```python
from build123d import *

# Parameters (mm, degrees)
BOSS_EXTRUDE1_DEPTH  = 3.175
BOSS_EXTRUDE2_DEPTH  = 3.175
M4_CLEARANCE_HOLE1_D = 4.5
SKETCH7_R            = 1.7
CUT_EXTRUDE1_DEPTH   = 4.175


with BuildPart() as part:
    # Sketch1 → Boss-Extrude1 (new body)
    with BuildSketch(Plane(origin=(0, 0, 0), x_dir=(1, 0, 0), z_dir=(0, 1, 0))):
        with BuildLine():
            ThreePointArc((0, 85), (-61.668691787, 60.61327124), (-89.979209979, 0.644490644))
            Line((-89.979209979, 0.644490644), (-69.92561449, 0.644490644))
            ThreePointArc((-69.92561449, 0.644490644), (-47.516373878, 46.462349638), (0, 65))
            Line((0, 65), (0, 85))
        make_face()
    extrude(amount=BOSS_EXTRUDE1_DEPTH)

    # Sketch2 → Boss-Extrude2 (add)
    with BuildSketch(Plane(origin=(0, 3.175, 0), x_dir=(1, 0, 0), z_dir=(0, 1, 0))):
        with BuildLine():
            Line((-89.979209979, 20.644490644), (-89.979209979, 0.644490644))
            ThreePointArc((-89.979209979, 0.644490644), (-88.75145348, 10.745821604), (-86.393355856, 20.644490644))
            Line((-86.393355856, 20.644490644), (-89.979209979, 20.644490644))
        make_face()
        with BuildLine():
            Line((-35, 85), (-35, 77.929830117))
            ThreePointArc((-35, 77.929830117), (-17.853482169, 83.214784737), (0, 85))
            Line((0, 85), (-35, 85))
        make_face()
    extrude(amount=-BOSS_EXTRUDE2_DEPTH)

    # M4 Clearance Hole1 (through all)
    with Locations(Plane.XZ):
        with Locations((-27.5, -70), (-7.5, -80), (-27.5, -80), (-7.5, -70)):
            Hole(M4_CLEARANCE_HOLE1_D / 2)

    # Sketch7 → Cut-Extrude1 (cut, through all)
    with BuildSketch(Plane.XZ):
        with Locations((-70.979209979, -15.644490644)):
            Circle(SKETCH7_R)
        with Locations((-85.979209979, -15.644490644)):
            Circle(SKETCH7_R)
        with Locations((-85.979209979, -5.644490644)):
            Circle(SKETCH7_R)
        with Locations((-70.979209979, -5.644490644)):
            Circle(SKETCH7_R)
    extrude(amount=-CUT_EXTRUDE1_DEPTH, mode=Mode.SUBTRACT)


solid = part.part
```
Source: CAD feature listing. Evaluate the final solid. Frame: model axes, mm. A direction names the side the tool comes from. Give positions to 0.01 mm unless a question says otherwise; leave off trailing zeros. Order: outer loops, then holes, each group sorted by start corner. A loop starts at its lowest first (then second) coordinate and runs counter-clockwise, first axis right, second up. Notation, with made-up numbers: (69.25, 42) -> (107.25, 42) arc R19 cw to (107.25, 64) -> close; hole circle Ø8 at (27.5, 55). An arc over 180 degrees is marked (long way). Use a Markdown table: item, result.
Q1. Access query for faces 4 (the face through (-88, 2, -20.644)), 5 (the face through (-17, 2, -85)). Directions: +Z, -Z, +X, -X, +Y, -Y. A direction counts if a zero-diameter tool reaches every point of the face in a straight line with its end or side. Return the directions, or none.
A:
| item | result |
|---|---|
| face 4 | -Z, -X, +Y, -Y |
| face 5 | -Z, +X, -X, +Y, -Y |
Q2. Section A-A (z = -80). Return the cut outline in (x, y) (3 decimals), and give its area (4 significant figures).
A:
| item | result |
|---|---|
| outline | (-35, 0) -> (-29.75, 0) -> (-29.75, 3.175) -> (-35, 3.175) -> close; (-25.25, 0) -> (-9.75, 0) -> (-9.75, 3.175) -> (-25.25, 3.175) -> close; (-5.25, 0) -> (0, 0) -> (0, 3.175) -> (-5.25, 3.175) -> close |
| area | 82.55 mm^2 |
Q3. Pull-direction query (X, two-part tool) for faces 1 (the face through (-69.36, 1.57, -15.13)), 2 (the face through (-69.717, 1.565, -2.761)), 3 (the face through (-35, 2, -82)); classes: +X half, -X half, draft (parallel to the pull), parting line (faces both ways), or undercut.
A:
| item | result |
|---|---|
| face 1 | undercut |
| face 2 | +X half |
| face 3 | -X half |
Q4. Section D-D (x = -45.5). Return the cut outline in (y, z) (3 decimals), and give its area (3 significant figures).
A:
| item | result |
|---|---|
| outline | (0, -72.678) -> (3.175, -72.678) -> (3.175, -48.248) -> (0, -48.248) -> close |
| area | 77.6 mm^2 |
Q5. Material intervals for line 1 (Z direction, x = -7.5, y = 1.4); line 2 (X direction, y = 1.05, z = -71.5); line 3 (Z direction, x = -70, y = 1.85), sorted ascending. Write a range as [from, to].
A:
| item | result |
|---|---|
| line 1 | [-85, -82.25], [-77.75, -72.25], [-67.75, -64.6] |
| line 2 | [-47.46, -29.18], [-25.82, -9.18], [-5.82, 0] |
| line 3 | [-51.67, -17.03], [-14.25, -7.03], [-4.25, -0.64] |
Q6. Section C-C (y = 1.55). Return the cut outline in (x, z), and give its area (3 significant figures).
A:
| item | result |
|---|---|
| outline | (-89.98, -20.64) -> (-86.39, -20.64) arc R90.17 ccw to (-35, -77.93) -> (-35, -85) -> (0, -85) -> (0, -65) arc R70.17 cw to (-69.29, -5.87) arc R1.7 cw (long way) to (-69.44, -4.93) arc R70.17 cw to (-69.93, -0.64) -> (-89.98, -0.64) -> close; hole circle Ø3.4 at (-85.98, -15.64); hole circle Ø3.4 at (-85.98, -5.64); hole circle Ø3.4 at (-70.98, -15.64); hole circle Ø4.5 at (-27.5, -80); hole circle Ø4.5 at (-27.5, -70); hole circle Ø4.5 at (-7.5, -80); hole circle Ø4.5 at (-7.5, -70) |
| area | 2,410 mm^2 |
Q7. First-contact query: P1, Ø2.5, axis at x = -70.98, z = -15.64, coming from the +Y side; P2, Ø1.5, axis at x = -42.5, y = 1.5, coming from the -Z side; P3, Ø1, axis at y = 2, z = -81, coming from the -X side. Flat tips, straight axial feed; report the tip coordinate or a pass-through.
A:
| item | result |
|---|---|
| P1 | through |
| P2 | z = -74.75 |
| P3 | x = -35 |
Q8. Section B-B (x = -7.5). Return the cut outline in (y, z) (3 decimals).
A:
| item | result |
|---|---|
| outline | (0, -85) -> (3.175, -85) -> (3.175, -82.25) -> (0, -82.25) -> close; (0, -77.75) -> (3.175, -77.75) -> (3.175, -72.25) -> (0, -72.25) -> close; (0, -67.75) -> (3.175, -67.75) -> (3.175, -64.598) -> (0, -64.598) -> close |
